from build123d import *

# Parameters (mm, degrees)
SKETCH_1_W          = 38.5
SKETCH_1_H          = 82
EXTRUDE_1_DEPTH     = 2
SKETCH_2_R          = 1.6
CUT_EXTRUDE_1_DEPTH = 2
SKETCH_3_W          = 3
SKETCH_3_H          = 69
SKETCH_3_W_2        = 26.5
SKETCH_3_H_2        = 74
CUT_EXTRUDE_2_DEPTH = 10
EXTRUDE_1_2_DEPTH   = 2
FILLET_1_R          = 2
FILLET_2_R          = 1.5


with BuildPart() as part:
    # 草图1 → Extrude 1 (new body)
    with BuildSketch(Plane(origin=(0, 0, 0), x_dir=(1, 0, 0), z_dir=(0, 1, 0))):
        Rectangle(SKETCH_1_W, SKETCH_1_H)
    extrude(amount=EXTRUDE_1_DEPTH)

    # 草图2 → 切除-拉伸1 (cut)
    with BuildSketch(Plane.XZ):
        with Locations(Location((16.25, -34, 0), (0, 0, 270))):
            Circle(SKETCH_2_R)
        with Locations(Location((16.25, 34, 0), (0, 0, 270))):
            Circle(SKETCH_2_R)
        with Locations(Location((-16.25, 34, 0), (0, 0, 270))):
            Circle(SKETCH_2_R)
    extrude(amount=-CUT_EXTRUDE_1_DEPTH, mode=Mode.SUBTRACT)

    # 草图3 → 切除-拉伸2 (cut)
    with BuildSketch(Plane.XZ):
        with Locations((-17.75, -6.5)):
            Rectangle(SKETCH_3_W, SKETCH_3_H)
        Rectangle(SKETCH_3_W_2, SKETCH_3_H_2)
    extrude(amount=-CUT_EXTRUDE_2_DEPTH, mode=Mode.SUBTRACT)

    # 草图4 → Extrude 1 2 (add)
    with BuildSketch(Plane.XZ):
        Polygon((-14.272000233, 35.90204029), (11.048434944, 12.333333333), (-15.451565056, -12.333333333), (12.227999767, -38.09795971), (14.272000233, -35.90204029), (-11.048434944, -12.333333333), (15.451565056, 12.333333333), (-12.227999767, 38.09795971), align=None)
        Polygon((12.227999767, 38.09795971), (-15.451565056, 12.333333333), (11.048434944, -12.333333333), (-14.272000233, -35.90204029), (-12.227999767, -38.09795971), (15.451565056, -12.333333333), (-11.048434944, 12.333333333), (14.272000233, 35.90204029), align=None)
    extrude(amount=-EXTRUDE_1_2_DEPTH)

    # 圆角1
    fillet_1_edges = [part.edges().sort_by_distance(p)[0] for p in [
        (-2.201565056, 1, 24.666666667),
        (-2.201565056, 1, 0),
        (-2.201565056, 1, -24.666666667),
        (0, 1, 26.715922191),
        (2.201565056, 1, -24.666666667),
        (2.201565056, 1, 0),
        (2.201565056, 1, 24.666666667),
        (0, 1, -26.715922191),
        (0, 1, 2.049255524),
        (0, 1, 22.617411143),
        (11.048434944, 1, 12.333333333),
        (0, 1, -2.049255524),
        (0, 1, -22.617411143),
        (-11.048434944, 1, -12.333333333),
        (11.048434944, 1, -12.333333333),
        (-11.048434944, 1, 12.333333333),
        (-11.048434944, 1, -37),
        (11.048434944, 1, -37),
        (13.25, 1, 34.950744476),
        (13.25, 1, -10.284077809),
        (13.25, 1, -14.382588857),
        (13.25, 1, -34.950744476),
        (13.25, 1, 10.284077809),
        (13.25, 1, 14.382588857),
        (11.048434944, 1, 37),
        (-11.048434944, 1, 37),
        (-13.25, 1, -34.950744476),
        (-13.25, 1, 10.284077809),
        (-13.25, 1, 14.382588857),
        (-13.25, 1, 34.950744476),
        (-13.25, 1, -10.284077809),
        (-13.25, 1, -14.382588857),
    ]]
    fillet(fillet_1_edges, radius=FILLET_1_R)

    # 圆角2
    fillet_2_edges = [part.edges().sort_by_distance(p)[0] for p in [
        (-16.25, 1, 28),
        (19.25, 1, -41),
        (19.25, 1, 41),
        (-19.25, 1, 41),
        (-19.25, 1, 28),
        (-16.25, 1, -41),
    ]]
    fillet(fillet_2_edges, radius=FILLET_2_R - 0.0001)  # a hair under: the kernel refuses the full size


solid = part.part
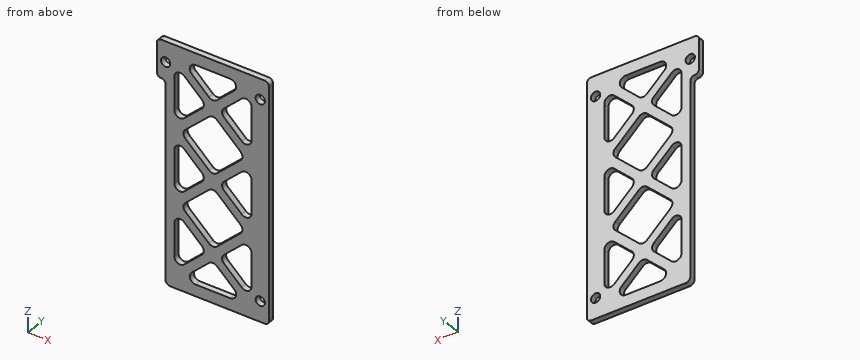
Can you work these out from the model? Positions are in its coordinate system, mm. Round coordinates to 2 decimals unless told otherwise and drop trailing zeros. Write each loop counter-clockwise with the first axis right and the second up, starting at its lowest first coordinate (ties: lowest second). Pieces come first, ordered by that corner, then holes. Notation, with made-up numbers: M 61,59 L 90,59 A6 cw 90,64 Z; hole C 51,59.25 d5. An arc over 180 degrees is marked long. Use CSV: the item, a comma, the result in double quotes.
(1) Imagine slicing it at A-A (x = 16.25). Write out the boundary of the cut face in (y, z).
Check values:
outline,"M 0,-41 L 2,-41 L 2,-35.6 L 0,-35.6 Z; M 0,-32.4 L 2,-32.4 L 2,32.4 L 0,32.4 Z; M 0,35.6 L 2,35.6 L 2,41 L 0,41 Z"
(2) I'm going to push flat-ended pins straight in: pin 1 (1.9 mm diameter, centred on x = 16.25, z = -34, fed in from -Y); pin 2 (1 mm diameter, centred on y = 1.5, z = 24, fed in from -X). Where does each tip first touch, or does it pass through?
Check values:
pin 1,"through"
pin 2,"x = -16.25"
(3) I need wall thicknesses on line 1 along X through (y, z) = (0.8, -30); line 2 along X through (y, z) = (1.5, -34); line 3 along X through (y, z) = (0.55, 34). Which ranges of each line are inside material? Lowest first, please.
Check values:
line 1,"-16.25 to -13.25, -7.93 to -3.53, 3.53 to 7.93, 13.25 to 19.25"
line 2,"-16.25 to -7.7, 7.7 to 14.65, 17.85 to 19.25"
line 3,"-19.25 to -17.85, -14.65 to -7.7, 7.7 to 14.65, 17.85 to 19.25"
(4) Imagine slicing it at C-C (z = 12.5). Write out the boundary of the cut face in (x, y), plus the area to 3 significant figures.
Check values:
outline,"M -16.25,0 L -10.11,0 L -10.11,2 L -16.25,2 Z; M 10.11,0 L 19.25,0 L 19.25,2 L 10.11,2 Z"
area,"30.6 mm^2"
(5) Imagine slicing it at B-B (x = -12.5). Write out the boundary of the cut face in (y, z), plus the area to 3 significant figures.
Check values:
outline,"M 0,-41 L 2,-41 L 2,-31.92 L 0,-31.92 Z; M 0,-17.42 L 2,-17.42 L 2,-7.25 L 0,-7.25 Z; M 0,7.25 L 2,7.25 L 2,17.42 L 0,17.42 Z; M 0,31.92 L 2,31.92 L 2,41 L 0,41 Z"
area,"77.0 mm^2"
(6) Imagine slicing it at D-D (y = 1.2). Count the separate pieces of the cut face and the enclosed holes in it, plus the area to 3 significant figures.
Check values:
separate pieces,"1"
enclosed holes,"13"
area,"1,650 mm^2"
